Here's the drawing with two shaded views (mm, measured from the low corner). I have some questions. Coordinates: 2 decimals unless noted, no trailing zeros. Write each loop counter-clockwise with the first axis right and the second up, starting at its lowest first coordinate (ties: lowest second). Pieces come first, ordered by that corner, then holes. Notation, with made-up numbers: (24, 27.5) -> (42, 27.5) arc R6 ccw to (42, 33.5) -> close; hole circle Ø10 at (61.25, 62.5). An arc over 180 degrees is marked (long way). Use a Markdown table: item, result. Add a question column.
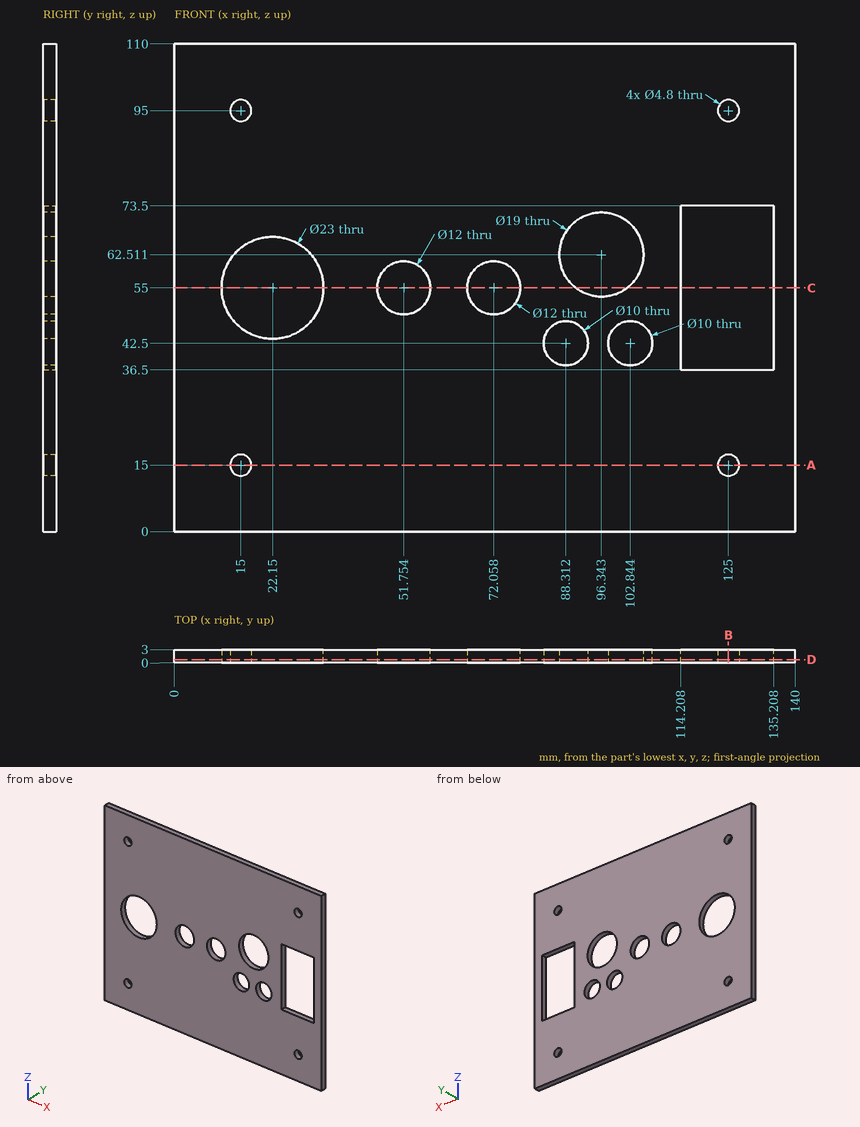
Q1. Suppose I cut it at C-C, the plane z = 55. Write out the boundary of the cut face in (x, y), and give its area (3 significant figures).
Q2. Please list where these lines run through material, in increasing order: line 1 (X direction, y = 1.45, z = 42.5); line 2 (Z direction, x = 125, y = 1.2); line 3 (X direction, y = 1, z = 95).
Q3. Suppose I cut it at A-A, the plane z = 15. Write out the boundary of the cut face in (x, y), and give its area (3 significant figures).
Q4. Suppose I cut it at B-B, the plane x = 125. Write out the boundary of the cut face in (y, z), and give its area (3 significant figures).
Q5. Suppose I cut it at D-D, the plane y = 0.75. State how many separate pieces and enclosed holes the cut face has, and give its area (3 significant figures).
Answer key:
| question | item | result |
|---|---|---|
| 1 | outline | (0, 0) -> (10.65, 0) -> (10.65, 3) -> (0, 3) -> close; (33.65, 0) -> (45.75, 0) -> (45.75, 3) -> (33.65, 3) -> close; (57.75, 0) -> (66.06, 0) -> (66.06, 3) -> (57.75, 3) -> close; (78.06, 0) -> (90.53, 0) -> (90.53, 3) -> (78.06, 3) -> close; (102.16, 0) -> (114.21, 0) -> (114.21, 3) -> (102.16, 3) -> close; (135.21, 0) -> (140, 0) -> (140, 3) -> (135.21, 3) -> close |
| 1 | area | 181 mm^2 |
| 2 | line 1 | x = 0 to 83.31, 93.31 to 97.84, 107.84 to 114.21, 135.21 to 140 |
| 2 | line 2 | z = 0 to 12.6, 17.4 to 36.5, 73.5 to 92.6, 97.4 to 110 |
| 2 | line 3 | x = 0 to 12.6, 17.4 to 122.6, 127.4 to 140 |
| 3 | outline | (0, 0) -> (12.6, 0) -> (12.6, 3) -> (0, 3) -> close; (17.4, 0) -> (122.6, 0) -> (122.6, 3) -> (17.4, 3) -> close; (127.4, 0) -> (140, 0) -> (140, 3) -> (127.4, 3) -> close |
| 3 | area | 391 mm^2 |
| 4 | outline | (0, 0) -> (3, 0) -> (3, 12.6) -> (0, 12.6) -> close; (0, 17.4) -> (3, 17.4) -> (3, 36.5) -> (0, 36.5) -> close; (0, 73.5) -> (3, 73.5) -> (3, 92.6) -> (0, 92.6) -> close; (0, 97.4) -> (3, 97.4) -> (3, 110) -> (0, 110) -> close |
| 4 | area | 190 mm^2 |
| 5 | separate pieces | 1 |
| 5 | enclosed holes | 11 |
| 5 | area | 13,500 mm^2 |
